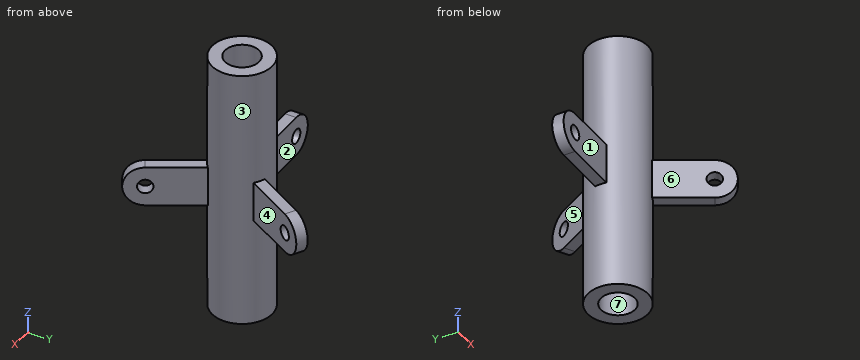
```python
from build123d import *

# Parameters (mm, degrees)
F0_R            = 10.6
F1_DEPTH        = 92
F2_R            = 6
F3_DEPTH        = 98.1
F5_DEPTH        = 2
F5_COPIES_COUNT = 3
F7_R            = 2.5
F8_DEPTH        = 4
F9_R            = 2.5
F10_DEPTH       = 4
F11_R           = 2.5
F12_DEPTH       = 4


# Not quite as in the source:
# - a feature of the source that left no trace in its solid (it failed there, or was rolled back) is left out
# - a pattern or mirror of a feature is missing from the dataset's text; its kind, count and spacing are read off the source's solid


with BuildPart() as f1:
    # F0 (on Top) → F1 (new body)
    with BuildSketch(Plane.XY):
        Circle(F0_R)
    extrude(amount=F1_DEPTH)

    # F2 (on face) → F3 (cut)
    with BuildSketch(Plane(origin=(0, 0, 0), x_dir=(1, 0, 0), z_dir=(0, 0, -1))):
        Circle(F2_R)
    extrude(amount=-F3_DEPTH, mode=Mode.SUBTRACT)

    # F4 (on Front) → F5 (join, symmetric)
    with BuildSketch(Plane.XZ):
        with BuildLine():
            Line((-9.7803492099, 52), (-29.4, 52))
            ThreePointArc((-29.4, 52), (-36.4, 45), (-29.4, 38))
            Line((-29.4, 38), (-9.7803492099, 38))
            Line((-9.7803492099, 38), (-9.7803492099, 52))
        make_face()
    f5 = extrude(amount=F5_DEPTH, both=True)

    # F5_copies: F5 ×3 about axis
    f5_copies_axis = Axis((0, 0, 0), (0, 0, 1))
    for i in range(1, F5_COPIES_COUNT):
        add(f5.rotate(f5_copies_axis, i * 360 / F5_COPIES_COUNT))

    # F7 (on face) → F8 (cut, through all)
    with BuildSketch(Plane.XZ.offset(2)):
        with Locations((-29.4, 45)):
            Circle(F7_R)
    extrude(amount=-F8_DEPTH, mode=Mode.SUBTRACT)

    # F9 (on face) → F10 (cut, through all)
    with BuildSketch(Plane(origin=(-1.7320508076, -1, 0), x_dir=(0.5, -0.8660254038, 0), z_dir=(-0.8660254038, -0.5, 0))):
        with Locations((29.4, 45)):
            Circle(F9_R)
    extrude(amount=-F10_DEPTH, mode=Mode.SUBTRACT)

    # F11 (on face) → F12 (cut, through all)
    with BuildSketch(Plane(origin=(1.7320508076, -1, 0), x_dir=(0.5, 0.8660254038, 0), z_dir=(0.8660254038, -0.5, 0))):
        with Locations((29.4, 45)):
            Circle(F11_R)
    extrude(amount=-F12_DEPTH, mode=Mode.SUBTRACT)


solid = f1.part
```
For this review, take the finished solid that the model builds, in its own axes (mm). Face numbers are marked on the shaded views. A direction names the side the tool comes from. Coordinates: 2 decimals unless noted, no trailing zeros. Write each loop counter-clockwise with the first axis right and the second up, starting at its lowest first coordinate (ties: lowest second). Pieces come first, ordered by that corner, then holes. Notation, with made-up numbers: (-39.75, 65.5) -> (-7.75, 65.5) arc R22 cw to (-7.75, 86.5) -> close; hole circle Ø8 at (-22, 63). An arc over 180 degrees is marked (long way). Put each result on its own line as item: value.
Q1. Take a section at A-A, the plane y = 0. State the section outline as (x, z) points.
From the geometry:
outline: (-29.4, 38) -> (-10.6, 38) -> (-10.6, 0) -> (-6, 0) -> (-6, 92) -> (-10.6, 92) -> (-10.6, 52) -> (-29.4, 52) arc R7 ccw to start; (6, 0) -> (10.6, 0) -> (10.6, 92) -> (6, 92) -> close; hole circle Ø5 at (-29.4, 45)
Q2. Take a section at D-D, the plane x = 8.5. State the section outline as (y, z) points.
From the geometry:
outline: (-18.72, 38) -> (-10.72, 38) -> (-10.72, 52) -> (-18.72, 52) -> close; (-6.33, 0) -> (6.33, 0) -> (6.33, 92) -> (-6.33, 92) -> close; (10.72, 38) -> (18.72, 38) -> (18.72, 52) -> (10.72, 52) -> close
Q3. Take a section at B-B, the plane x = 0. State the section outline as (y, z) points, then the cut area to 3 significant figures.
From the geometry:
outline: (-10.6, 0) -> (-6, 0) -> (-6, 92) -> (-10.6, 92) -> close; (6, 0) -> (10.6, 0) -> (10.6, 92) -> (6, 92) -> close
area: 846 mm2
Q4. Take a section at C-C, the plane z = 45. State the section outline as (x, y) points.
From the geometry:
outline: (-36.4, -2) -> (-31.9, -2) -> (-31.9, 2) -> (-36.4, 2) -> close; (-26.9, -2) -> (-10.41, -2) arc R10.6 ccw to (3.47, -10.01) -> (11.72, -24.3) -> (15.18, -22.3) -> (6.94, -8.01) arc R10.6 ccw to (6.94, 8.01) -> (15.18, 22.3) -> (11.72, 24.3) -> (3.47, 10.01) arc R10.6 ccw to (-10.41, 2) -> (-26.9, 2) -> close; (14.22, -28.63) -> (16.47, -32.52) -> (19.93, -30.52) -> (17.68, -26.63) -> close; (14.22, 28.63) -> (17.68, 26.63) -> (19.93, 30.52) -> (16.47, 32.52) -> close; hole circle Ø12 at (0, 0)
Q5. Clearance check with flat-ended pins moving along their axes: pin 1 Ø4 at (x, y) = (9, -16.5) entering from -Z; pin 2 Ø12 at (x, y) = (10, 8.5) entering from -Z; pin 3 Ø11 at (x, z) = (-25.5, 46.5) entering from -Y; pin 4 Ø4 at (x, z) = (10, 53) entering from +Y. State where each tip first meets the part, or that it passes through.
From the geometry:
pin 1: stops at z = 38
pin 2: stops at z = 0
pin 3: stops at y = -2
pin 4: stops at y = 24.32
Q6. Wall thickness on L1, parallel to X at y = 0, z = 57; L2, parallel to Z at x = -29, y = 0; L3, parallel to X at y = 0, z = 47: over which ranges is each line inside the solid? List them lowest first.
From the geometry:
L1: x = -10.6 to -6, 6 to 10.6
L2: z = 38 to 42.53, 47.47 to 52
L3: x = -36.11 to -30.9, -27.9 to -6, 6 to 10.6
Q7. The part is to be moulded in two halves that separate along Y. For the marked faces 5, 6 and 7, say which applies: +Y half, -Y half, draft (parallel to the pull), parting line (faces both ways), or undercut.
From the geometry:
face 5: +Y half
face 6: -Y half
face 7: undercut
Q8. Tool access review of the marked faces 1, 2, 3 and 4: name each direction out of +Z, -Z, +X, -X, +Y, -Y from which nothing blocks a thin tool from reaching the whole face with its end or side.
From the geometry:
face 1: +Z, -Z, -X, -Y
face 2: +Z, -Z, -X, +Y
face 3: none
face 4: +Z, -Z, +X
